Source: CAD feature listing. Evaluate the final solid. Frame: model axes, mm. Round coordinates to 2 decimals unless told otherwise and drop trailing zeros. Loops run counter-clockwise (first coordinate to the right, second up) from the corner with the lowest first, then second, coordinate; pieces in that order, holes last. Notation, with made-up numbers: (31.25, 33) - (80.25, 33) arc R5 cw to (80.25, 42) - close; hole circle Ø6 at (-6, -28.75). An arc over 180 degrees is marked (long way). One line per question, with ' | ' between items. Start each with the question number.
1. Pin query (flat end, axial travel): pin 1 (5 mm diameter, centred on y = 501, z = 2.5, fed in from -X); pin 2 (11 mm diameter, centred on x = 494.38, y = 94.2, fed in from -Z); pin 3 (3 mm diameter, centred on x = 809, z = 6, fed in from +Y); pin 4 (3 mm diameter, centred on y = 285.5, z = 4.5, fed in from +X). Return the tip coordinate at first contact, or that it passes through.
2. Cut plane A-A (x = 317.5). Return loops of the section in (y, z), then the cut area to 3 significant figures.
3. Cut plane B-B (z = 5). State how many separate pieces and enclosed holes the cut face has, then the cut area to 3 significant figures.
4. Ray query, line 1 (X direction, y = 380, z = 4.5); line 2 (Y direction, x = 640, z = 5.25); line 3 (Y direction, x = 459.5, z = 5). Return the intervals inside material, ascending.
```python
from build123d import *

# Parameters (mm, degrees)
ESQUISSE1_W             = 880
ESQUISSE1_H             = 530
ESQUISSE1_R             = 121
ESQUISSE1_R_2           = 6.75
BOSS_EXTRU_1_DEPTH      = 10
CHANFREIN1_SIZE         = 80
ESQUISSE2_W             = 100
ESQUISSE2_H             = 10
ESQUISSE2_W_2           = 80
ESQUISSE2_H_2           = 40
ENL_V_MAT_EXTRU_1_DEPTH = 10


with BuildPart() as part:
    # Esquisse1 → Boss.-Extru.1 (new body)
    with BuildSketch(Plane.XY):
        with Locations((440, 265)):
            Rectangle(ESQUISSE1_W, ESQUISSE1_H)
        with Locations((640, 200)):
            Circle(ESQUISSE1_R, mode=Mode.SUBTRACT)
        with Locations((820, 200)):
            Circle(ESQUISSE1_R_2, mode=Mode.SUBTRACT)
        with Locations((811.190172933, 144.376941013)):
            Circle(ESQUISSE1_R_2, mode=Mode.SUBTRACT)
        with Locations((785.623058987, 94.198654587)):
            Circle(ESQUISSE1_R_2, mode=Mode.SUBTRACT)
        with Locations((745.801345413, 54.376941013)):
            Circle(ESQUISSE1_R_2, mode=Mode.SUBTRACT)
        with Locations((695.623058987, 28.809827067)):
            Circle(ESQUISSE1_R_2, mode=Mode.SUBTRACT)
        with Locations((640, 20)):
            Circle(ESQUISSE1_R_2, mode=Mode.SUBTRACT)
        with Locations((584.376941012, 28.809827067)):
            Circle(ESQUISSE1_R_2, mode=Mode.SUBTRACT)
        with Locations((534.198654587, 54.376941013)):
            Circle(ESQUISSE1_R_2, mode=Mode.SUBTRACT)
        with Locations((494.376941012, 94.198654587)):
            Circle(ESQUISSE1_R_2, mode=Mode.SUBTRACT)
        with Locations((468.809827067, 144.376941013)):
            Circle(ESQUISSE1_R_2, mode=Mode.SUBTRACT)
        with Locations((460, 200)):
            Circle(ESQUISSE1_R_2, mode=Mode.SUBTRACT)
        with Locations((468.809827067, 255.623058987)):
            Circle(ESQUISSE1_R_2, mode=Mode.SUBTRACT)
        with Locations((494.376941012, 305.801345413)):
            Circle(ESQUISSE1_R_2, mode=Mode.SUBTRACT)
        with Locations((534.198654587, 345.623058987)):
            Circle(ESQUISSE1_R_2, mode=Mode.SUBTRACT)
        with Locations((584.376941012, 371.190172933)):
            Circle(ESQUISSE1_R_2, mode=Mode.SUBTRACT)
        with Locations((640, 380)):
            Circle(ESQUISSE1_R_2, mode=Mode.SUBTRACT)
        with Locations((695.623058987, 371.190172933)):
            Circle(ESQUISSE1_R_2, mode=Mode.SUBTRACT)
        with Locations((745.801345413, 345.623058987)):
            Circle(ESQUISSE1_R_2, mode=Mode.SUBTRACT)
        with Locations((785.623058987, 305.801345413)):
            Circle(ESQUISSE1_R_2, mode=Mode.SUBTRACT)
        with Locations((811.190172933, 255.623058987)):
            Circle(ESQUISSE1_R_2, mode=Mode.SUBTRACT)
        with Locations(Location((68.809827067, 255.623058987, 0), (0, 0, 180))):
            Circle(ESQUISSE1_R_2, mode=Mode.SUBTRACT)
        with Locations(Location((94.376941013, 305.801345413, 0), (0, 0, 180))):
            Circle(ESQUISSE1_R_2, mode=Mode.SUBTRACT)
        with Locations(Location((134.198654587, 345.623058987, 0), (0, 0, 180))):
            Circle(ESQUISSE1_R_2, mode=Mode.SUBTRACT)
        with Locations(Location((184.376941013, 371.190172933, 0), (0, 0, 180))):
            Circle(ESQUISSE1_R_2, mode=Mode.SUBTRACT)
        with Locations(Location((240, 380, 0), (0, 0, 180))):
            Circle(ESQUISSE1_R_2, mode=Mode.SUBTRACT)
        with Locations(Location((295.623058987, 371.190172933, 0), (0, 0, 180))):
            Circle(ESQUISSE1_R_2, mode=Mode.SUBTRACT)
        with Locations(Location((345.801345413, 345.623058987, 0), (0, 0, 180))):
            Circle(ESQUISSE1_R_2, mode=Mode.SUBTRACT)
        with Locations(Location((385.623058987, 305.801345413, 0), (0, 0, 180))):
            Circle(ESQUISSE1_R_2, mode=Mode.SUBTRACT)
        with Locations(Location((411.190172933, 255.623058987, 0), (0, 0, 180))):
            Circle(ESQUISSE1_R_2, mode=Mode.SUBTRACT)
        with Locations(Location((420, 200, 0), (0, 0, 180))):
            Circle(ESQUISSE1_R_2, mode=Mode.SUBTRACT)
        with Locations(Location((411.190172933, 144.376941013, 0), (0, 0, 180))):
            Circle(ESQUISSE1_R_2, mode=Mode.SUBTRACT)
        with Locations(Location((385.623058987, 94.198654587, 0), (0, 0, 180))):
            Circle(ESQUISSE1_R_2, mode=Mode.SUBTRACT)
        with Locations(Location((345.801345413, 54.376941013, 0), (0, 0, 180))):
            Circle(ESQUISSE1_R_2, mode=Mode.SUBTRACT)
        with Locations(Location((295.623058987, 28.809827067, 0), (0, 0, 180))):
            Circle(ESQUISSE1_R_2, mode=Mode.SUBTRACT)
        with Locations(Location((240, 20, 0), (0, 0, 180))):
            Circle(ESQUISSE1_R_2, mode=Mode.SUBTRACT)
        with Locations(Location((184.376941013, 28.809827067, 0), (0, 0, 180))):
            Circle(ESQUISSE1_R_2, mode=Mode.SUBTRACT)
        with Locations(Location((134.198654587, 54.376941013, 0), (0, 0, 180))):
            Circle(ESQUISSE1_R_2, mode=Mode.SUBTRACT)
        with Locations(Location((94.376941013, 94.198654587, 0), (0, 0, 180))):
            Circle(ESQUISSE1_R_2, mode=Mode.SUBTRACT)
        with Locations(Location((68.809827067, 144.376941013, 0), (0, 0, 180))):
            Circle(ESQUISSE1_R_2, mode=Mode.SUBTRACT)
        with Locations(Location((60, 200, 0), (0, 0, 180))):
            Circle(ESQUISSE1_R_2, mode=Mode.SUBTRACT)
        with Locations(Location((240, 200, 0), (0, 0, 180))):
            Circle(ESQUISSE1_R, mode=Mode.SUBTRACT)
    extrude(amount=BOSS_EXTRU_1_DEPTH)

    # Chanfrein1
    chanfrein1_edges = [part.edges().sort_by_distance(p)[0] for p in [
        (880, 0, 5),
        (0, 0, 5),
    ]]
    chamfer(chanfrein1_edges, length=CHANFREIN1_SIZE)

    # Esquisse2 → Enlèv. mat.-Extru.1 (cut)
    with BuildSketch(Plane(origin=(0, 0, 0), x_dir=(-1, 0, 0), z_dir=(0, 0, -1))):
        Polygon((-880, 530), (-840, 530), (-780, 530), (-780, 520), (-840, 520), (-840, 120), (-880, 120), align=None)
        with Locations((-570, 525)):
            Rectangle(ESQUISSE2_W, ESQUISSE2_H)
        with Locations((-310, 525)):
            Rectangle(ESQUISSE2_W, ESQUISSE2_H)
        Polygon((-100, 530), (-100, 520), (-40, 520), (-40, 120), (0, 120), (0, 530), (-40, 530), align=None)
        with Locations((-440, 500)):
            Rectangle(ESQUISSE2_W_2, ESQUISSE2_H_2)
    extrude(amount=-ENL_V_MAT_EXTRU_1_DEPTH, mode=Mode.SUBTRACT)


solid = part.part
```
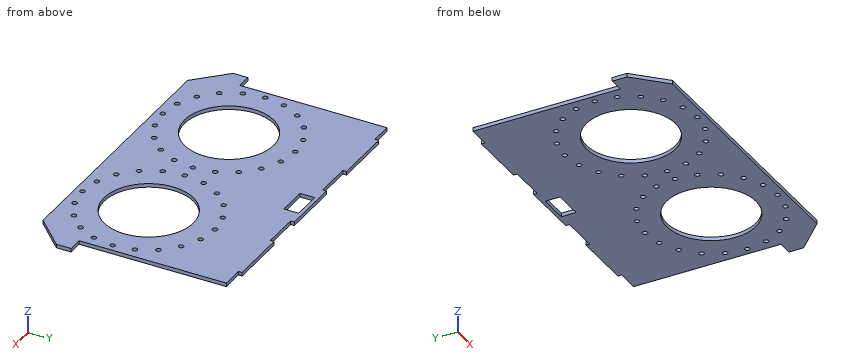
Answers follow:
1) pin 1: stops at x = 40 | pin 2: passes through | pin 3: stops at y = 520 | pin 4: stops at x = 840
2) outline: (0, 0) - (107.08, 0) - (107.08, 10) - (0, 10) - close; (292.92, 0) - (520, 0) - (520, 10) - (292.92, 10) - close | area: 3,340 mm2
3) separate pieces: 1 | enclosed holes: 43 | area: 323,000 mm2
4) line 1: x = 40 to 233.25, 246.75 to 633.25, 646.75 to 840 | line 2: y = 0 to 13.25, 26.75 to 79, 321 to 373.25, 386.75 to 530 | line 3: y = 0 to 193.27, 206.73 to 480, 520 to 530
